Autodesk Inventor part; units mm, degrees
ref_plane "YZ Plane" through (0, 0, 0) normal (1, 0, 0) x (0, 1, 0)
ref_plane "XZ Plane" through (0, 0, 0) normal (0, 1, 0) x (-1, 0, 0)
ref_plane "XY Plane" through (0, 0, 0) normal (0, 0, 1) x (1, 0, 0)
sketch "Sketch1" plane through (0, 0, 0) normal (0, 1, 0) x (-1, 0, 0)
  line L0 (71.1097, -38.0648) -> (71.1097, -13.0648)
  line L1 (71.1097, -13.0648) -> (74.1097, -13.0648)
  line L2 (74.1097, -13.0648) -> (74.1097, 11.9352)
  line L3 (74.1097, 11.9352) -> (71.1097, 11.9352)
  line L4 (71.1097, 11.9352) -> (71.1097, 36.9352)
  line L5 (-72.8903, -38.0648) -> (-72.8903, -13.0648)
  line L6 (-72.8903, 36.9352) -> (-72.8903, 11.9352)
  line L7 (-72.8903, -13.0648) -> (-75.8903, -13.0648)
  line L8 (-75.8903, -13.0648) -> (-75.8903, 11.9352)
  line L9 (-75.8903, 11.9352) -> (-72.8903, 11.9352)
  line L10 (71.1097, -38.0648) -> (-72.8903, -38.0648)
  line L11 (71.1097, 36.9352) -> (-72.8903, 36.9352)
  point P0 (0, 0)
extrude "Extrusion1" add sketch "Sketch1" along normal blind 3
sketch "Sketch2" plane through (0, 3, 0) normal (0, 1, 0) x (1, 0, 0)
  line L0 (-71.1097, -36.9352) -> (72.8903, -36.9352)
  line L1 (-66.1097, -31.9352) -> (-56.1097, -31.9352)
  line L2 (-56.1097, -31.9352) -> (-56.1097, -28.9352)
  line L3 (-56.1097, -28.9352) -> (-66.1097, -28.9352)
  line L4 (-66.1097, -28.9352) -> (-66.1097, -31.9352)
  line L5 (72.8903, 38.0648) -> (-71.1097, 38.0648)
  line L6 (-56.1097, 30.0648) -> (-66.1097, 30.0648)
  line L7 (-66.1097, 30.0648) -> (-66.1097, 33.0648)
  line L8 (-66.1097, 33.0648) -> (-56.1097, 33.0648)
  line L9 (-56.1097, 33.0648) -> (-56.1097, 30.0648)
  line L10 (67.8903, 33.0648) -> (57.8903, 33.0648)
  line L11 (57.8903, 33.0648) -> (57.8903, 30.0648)
  line L12 (57.8903, 30.0648) -> (67.8903, 30.0648)
  line L13 (67.8903, 30.0648) -> (67.8903, 33.0648)
  line L14 (67.8903, -31.9352) -> (57.8903, -31.9352)
  line L15 (57.8903, -31.9352) -> (57.8903, -28.9352)
  line L16 (57.8903, -28.9352) -> (67.8903, -28.9352)
  line L17 (67.8903, -28.9352) -> (67.8903, -31.9352)
  point P0 (0, 0)
extrude "Extrusion2" cut sketch "Sketch2" against normal blind 30
sketch "Sketch3" plane through (0, 3, 0) normal (0, 1, 0) x (1, 0, 0)
  line L0 (72.8903, 38.0648) -> (-71.1097, 38.0648)
  line L1 (-71.1097, -36.9352) -> (72.8903, -36.9352)
  line L2 (-74.1097, 13.0648) -> (-74.1097, -11.9352)
  line L3 (75.8903, -11.9352) -> (75.8903, 13.0648)
  circle A0 centre (6.2215, -7.0252) radius 2
  circle A1 centre (6.2215, 8.1548) radius 2
  line L4 (2.4888, 13.0648) -> (-12.5112, 13.0648)
  line L5 (-12.5112, 13.0648) -> (-12.5112, -11.9352)
  line L6 (-12.5112, -11.9352) -> (2.4888, -11.9352)
  line L7 (2.4888, -11.9352) -> (2.4888, 13.0648)
  line L8 (-58.6097, -9.9352) -> (-44.6097, -9.9352)
  line L9 (-44.6097, -9.9352) -> (-44.6097, 11.0648)
  line L10 (-44.6097, 11.0648) -> (-58.6097, 11.0648)
  line L11 (-58.6097, 11.0648) -> (-58.6097, -9.9352)
  line L12 (60.3903, 11.0648) -> (46.3903, 11.0648)
  line L13 (46.3903, 11.0648) -> (46.3903, -9.9352)
  line L14 (46.3903, -9.9352) -> (60.3903, -9.9352)
  line L15 (60.3903, -9.9352) -> (60.3903, 11.0648)
  line L16 (-71.1097, -36.9352) -> (72.8903, -36.9352)
  point P0 (0, 0)
  dimension "d56" = 14
  dimension "d57" = 21
  dimension "d59" = 25
  dimension "d60" = 15
  dimension "d61" = 4
  dimension "d62" = 4
  dimension "d63" = 14
  dimension "d64" = 21
extrude "Extrusion3" cut sketch "Sketch3" against normal blind 10
sketch "Sketch4" plane through (0, 3, 0) normal (0, 1, 0) x (1, 0, 0)
  line L0 (-56.1097, 33.0648) -> (-41.1097, 33.0648)
  line L1 (-41.1097, 33.0648) -> (-41.1097, 29.924)
  line L2 (-41.1097, 29.924) -> (-56.1097, 29.924)
  line L3 (-56.1097, 29.924) -> (-56.1097, 33.0648)
  line L4 (57.8903, 30.0648) -> (57.8903, 33.0648)
  line L5 (57.8903, 33.0648) -> (42.8903, 33.0648)
  line L6 (42.8903, 33.0648) -> (42.8903, 29.924)
  line L7 (42.8903, 29.924) -> (57.8903, 29.924)
  line L8 (57.8903, 29.924) -> (57.8903, 33.0648)
  line L9 (-56.1097, -31.9352) -> (-41.1097, -31.9352)
  line L10 (-41.1097, -31.9352) -> (-41.1097, -28.9352)
  line L11 (-41.1097, -28.9352) -> (-56.1097, -28.9352)
  line L12 (-56.1097, -28.9352) -> (-56.1097, -31.9352)
  line L13 (57.8903, -31.9352) -> (57.8903, -28.9352)
  line L14 (57.8903, -28.9352) -> (42.8903, -28.9352)
  line L15 (42.8903, -28.9352) -> (42.8903, -31.9352)
  line L16 (42.8903, -31.9352) -> (57.8903, -31.9352)
  line L17 (57.8903, -31.9352) -> (57.8903, -28.9352)
  point P0 (0, 0)
  dimension "d67" = 15
  dimension "d68" = 15
extrude "Extrusion4" cut sketch "Sketch4" against normal blind 10
sketch "Sketch5" plane through (-41.1097, 3, -29.924) normal (0, 0, -1) x (-1, 0, 0)
  line L0 (15, -3) -> (0, -3)
  line L1 (0, 0) -> (15, 0)
  line L2 (15, -3) -> (0, -3)
  line L3 (0, -3) -> (0, 0)
  line L4 (0, 0) -> (15, 0)
  line L5 (15, 0) -> (15, -3)
  point P0 (-41.1097, -3)
extrude "Extrusion5" add sketch "Sketch5" along normal blind 0.14
sketch "Sketch6" plane through (57.8903, 3, -29.924) normal (0, 0, -1) x (-1, 0, 0)
  line L0 (0, 0) -> (15, 0)
  line L1 (15, 0) -> (15, -3)
  line L2 (15, -3) -> (0, -3)
  line L3 (0, -3) -> (0, 0)
  point P0 (57.8903, -3)
extrude "Extrusion6" add sketch "Sketch6" along normal blind 0.14
properties part number "Level4 (Sensor + Schakelaar)"
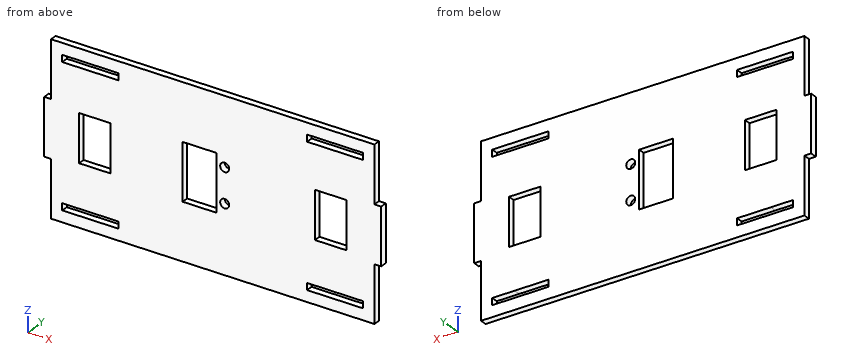
Part model, mm, in its own coordinate system. Round coordinates to 2 decimals unless told otherwise and drop trailing zeros. Order: outer loops, then holes, each group sorted by start corner. A loop starts at its lowest first (then second) coordinate and runs counter-clockwise, first axis right, second up. Notation, with made-up numbers: M 65,42 L 115,42 A25 cw 115,65 Z; hole C 60.5,61 d2. An arc over 180 degrees is marked long. Answer in a Markdown table with one row per item. Add a question column.
Q1. Cut at C-C on x = 64. Give the cut face in (y, z).
Q2. Cut at D-D on y = 1.3. Give the number of separate pieces and of enclosed holes in the cut face, and give its area (3 significant figures).
Q3. Pin check, flat tips, straight feed: pin 1 (0.9 mm diameter, centred on y = 1, z = 23, fed in from -X); pin 2 (1.5 mm diameter, centred on y = 1.5, z = 30, fed in from +X). Stop position of each tip, or through.
Q4. Wall check: L1, parallel to Z at x = 66, y = 2.35; L2, parallel to Z at x = -52.5, y = 2.15; L3, parallel to X at y = 0.45, z = 4.5. Give the ranges that are in metal, low to high. Write a range as from..to.
Q5. Cut at B-B on z = -1. Give the cut face in (x, y).
Q6. Cut at A-A on x = -47.5. Give the cut face in (y, z), and give its area (3 significant figures).
Established:
| question | item | result |
|---|---|---|
| 1 | outline | M 0,-38.06 L 3,-38.06 L 3,-33.06 L 0,-33.06 Z; M 0,-30.06 L 3,-30.06 L 3,28.94 L 0,28.94 Z; M 0,31.94 L 3,31.94 L 3,36.94 L 0,36.94 Z |
| 2 | separate pieces | 1 |
| 2 | enclosed holes | 9 |
| 2 | area | 9,660 mm2 |
| 3 | pin 1 | stops at x = -71.11 |
| 3 | pin 2 | stops at x = 72.89 |
| 4 | L1 | z = -38.06..-33.06, -30.06..28.94, 31.94..36.94 |
| 4 | L2 | z = -38.06..-33.06, -30.06..-11.06, 9.94..28.94, 31.94..36.94 |
| 4 | L3 | x = -74.11..-58.61, -44.61..-12.51, 2.49..46.39, 60.39..75.89 |
| 5 | outline | M -74.11,0 L -58.61,0 L -58.61,3 L -74.11,3 Z; M -44.61,0 L -12.51,0 L -12.51,3 L -44.61,3 Z; M 2.49,0 L 46.39,0 L 46.39,3 L 2.49,3 Z; M 60.39,0 L 75.89,0 L 75.89,3 L 60.39,3 Z |
| 6 | outline | M 0,-38.06 L 3,-38.06 L 3,-33.06 L 0,-33.06 Z; M 0,-30.06 L 3,-30.06 L 3,-11.06 L 0,-11.06 Z; M 0,9.94 L 3,9.94 L 3,28.94 L 0,28.94 Z; M 0,31.94 L 3,31.94 L 3,36.94 L 0,36.94 Z |
| 6 | area | 144 mm2 |
